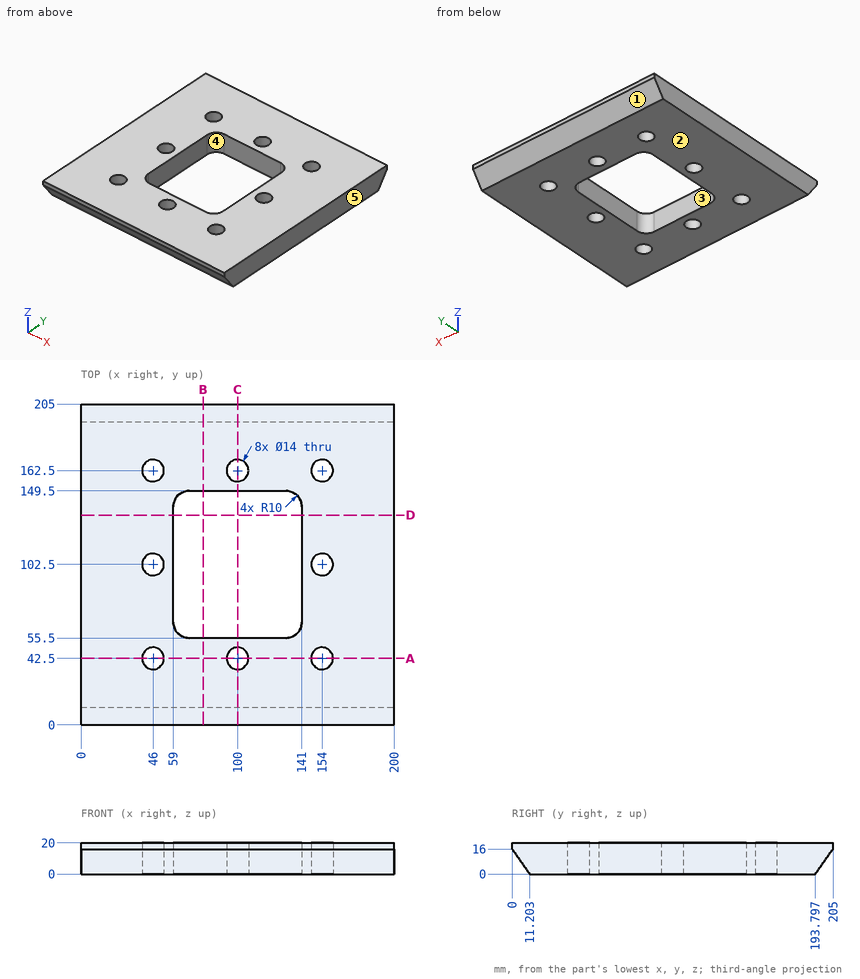
Here's the drawing with two shaded views (mm, measured from the low corner). I have some questions. A direction names the side the tool comes from. Give positions to 0.01 mm unless a question says otherwise; leave off trailing zeros. Order: outer loops, then holes, each group sorted by start corner. A loop starts at its lowest first (then second) coordinate and runs counter-clockwise, first axis right, second up. Notation, with made-up numbers: (-18.5, -18) -> (25.5, -18) arc R16 ccw to (25.5, -14) -> close; hole circle Ø2 at (39, 63.5). An arc over 180 degrees is marked (long way). One line per item, written item: value. Start each with the question number.
1. I need wall thicknesses on probe 1 along X at (y, z) = (139.5, 6); probe 2 along Y at (x, z) = (152.5, 6.75); probe 3 along Y at (x, z) = (44.5, 12.5). Which ranges of each line are inside material? Lowest first, please. Write a range as from..to.
2. Imagine slicing it at D-D, the plane y = 134. List the corners of the cut face in (x, z) for me, plus the area to 3 significant figures.
3. Imagine slicing it at A-A, the plane y = 42.5. List the corners of the cut face in (x, z) for me.
4. We'd pull the mould along Y, two halves only. Please class the marked faces 1, 2 and 3: released by +Y, released by -Y, zero draft, split by the parting line, or undercut.
5. Imagine slicing it at B-B, the plane x = 78. List the corners of the cut face in (y, z) for me.
6. Imagine slicing it at C-C, the plane x = 100. List the corners of the cut face in (y, z) for me, plus the area to 3 significant figures.
7. For the marked faces 4 and 5, which set-ups out of +Z, -Z, +X, -X, +Y, -Y let a thin tool reach every point of the face, with its end or its side?
8. Will these pins go through, and if not, where does the flat tip stop? pin 1 Ø6 at (x, z) = (110.5, 12) entering from -Y; pin 2 Ø4 at (x, z) = (165, 8.5) entering from +Y; pin 3 Ø1 at (x, z) = (78.5, 3) entering from +Y.
Values follow:
1. probe 1: x = 0..59, 141..200
1. probe 2: y = 6.48..35.66, 49.34..95.66, 109.34..155.66, 169.34..198.52
1. probe 3: y = 2.45..35.66, 49.34..95.66, 109.34..155.66, 169.34..202.55
2. outline: (0, 0) -> (59, 0) -> (59, 20) -> (0, 20) -> close; (141, 0) -> (200, 0) -> (200, 20) -> (141, 20) -> close
2. area: 2,360 mm2
3. outline: (0, 0) -> (39, 0) -> (39, 20) -> (0, 20) -> close; (53, 0) -> (93, 0) -> (93, 20) -> (53, 20) -> close; (107, 0) -> (147, 0) -> (147, 20) -> (107, 20) -> close; (161, 0) -> (200, 0) -> (200, 20) -> (161, 20) -> close
4. face 1: released by +Y
4. face 2: zero draft
4. face 3: undercut
5. outline: (0, 16) -> (11.2, 0) -> (55.5, 0) -> (55.5, 20) -> (0, 20) -> close; (149.5, 0) -> (193.8, 0) -> (205, 16) -> (205, 20) -> (149.5, 20) -> close
6. outline: (0, 16) -> (11.2, 0) -> (35.5, 0) -> (35.5, 20) -> (0, 20) -> close; (49.5, 0) -> (55.5, 0) -> (55.5, 20) -> (49.5, 20) -> close; (149.5, 0) -> (155.5, 0) -> (155.5, 20) -> (149.5, 20) -> close; (169.5, 0) -> (193.8, 0) -> (205, 16) -> (205, 20) -> (169.5, 20) -> close
6. area: 1,480 mm2
7. face 4: +Z, -Z
7. face 5: +Z, -Z, +X, +Y, -Y
8. pin 1: stops at y = 0.7
8. pin 2: stops at y = 201.15
8. pin 3: stops at y = 196.25
